from build123d import *

# Parameters (mm, degrees)
F2_R     = 4
F3_DEPTH = 12.5
F4_SIZE  = 1.99999


# Not quite as in the source:
# - a fillet or chamfer is up to 0.001 mm smaller than in the source, because OpenCascade refuses the exact size


with BuildPart() as f1:
    # F0 (on Top) → F1 (revolve)
    with BuildSketch(Plane.XY):
        Polygon((0, 6), (0, 0), (84, 0), (84, 12), (80, 12), (80, 6), align=None)
    revolve(axis=Axis((42, 0, 0), (1, 0, 0)))

    # F2 (on Top) → F3 (cut, symmetric)
    with BuildSketch(Plane.XY):
        with Locations((6, 0)):
            Circle(F2_R)
    extrude(amount=F3_DEPTH, both=True, mode=Mode.SUBTRACT)

    # F4 (size 2 in the source; OpenCascade refuses exactly that, so slightly less here)
    f4_edges = [f1.edges().sort_by_distance(p)[0] for p in [
        (0, -6, 0),
    ]]
    chamfer(f4_edges, length=F4_SIZE)


solid = f1.part
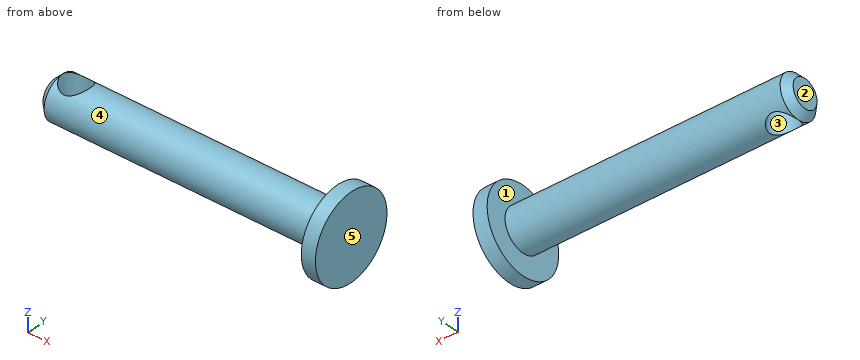
Geometry: final body of the model. Coordinates: model frame, mm. Face numbers are marked on the shaded views. A direction names the side the tool comes from. Round coordinates to 2 decimals unless told otherwise and drop trailing zeros. Order: outer loops, then holes, each group sorted by start corner. A loop starts at its lowest first (then second) coordinate and runs counter-clockwise, first axis right, second up.
Q1. Mould query, pull axis Y, two halves, no side actions, for the marked faces 3, 4 and 5. Classes: released by +Y, released by -Y, zero draft, split by the parting line, or undercut.
Result sheet:
face 3: undercut
face 4: split by the parting line
face 5: zero draft
Q2. Section C-C, the plane x = 66. Output: boundary loops of the cut face in (y, z), and give its area (3 significant figures).
Result sheet:
outline: circle Ø12 at (0, 0)
area: 113 mm2
Q3. Access query for the marked faces 1 and 2. Directions: +Z, -Z, +X, -X, +Y, -Y. A direction counts if a zero-diameter tool reaches every point of the face in a straight line with its end or side. Return the directions, or none.
Result sheet:
face 1: -X
face 2: +Z, -Z, -X, +Y, -Y
Q4. Section B-B, the plane z = 0. Output: boundary loops of the cut face in (x, y), and give its area (3 significant figures).
Result sheet:
outline: (0, -4) - (2, -6) - (80, -6) - (80, -12) - (84, -12) - (84, 12) - (80, 12) - (80, 6) - (2, 6) - (0, 4) - close; hole circle Ø8 at (6, 0)
area: 1,000 mm2
Q5. Section D-D, the plane x = 6. Output: boundary loops of the cut face in (y, z), and give its area (3 significant figures).
Result sheet:
outline: (-4, -4.47) - (-4, 4.47) arc R6 ccw to start; (4, -4.47) arc R6 ccw to (4, 4.47) - close
area: 24.8 mm2
Q6. Pin query (flat end, axial travel): pin 1 (9 mm diameter, centred on x = 6, y = 0, fed in from -Z); pin 2 (2 mm diameter, centred on x = 66.5, z = 2, fed in from -Y); pin 3 (12 mm diameter, centred on x = 37.5, y = -3.5, fed in from +Z). Return the tip coordinate at first contact, or that it passes through.
Result sheet:
pin 1: stops at z = -6
pin 2: stops at y = -5.92
pin 3: stops at z = 6
Q7. Material intervals for probe 1 along X at (y, z) = (0, 2); probe 2 along X at (y, z) = (10.5, -2.25); probe 3 along Y at (x, z) = (6, -1), sorted ascending.
Result sheet:
probe 1: x = 0 to 2, 10 to 84
probe 2: x = 80 to 84
probe 3: y = -5.92 to -4, 4 to 5.92
